Read the model definition and answer for the solid it produces. Units are mm, in the model's axes. A direction names the side the tool comes from. Coordinates: 2 decimals unless noted, no trailing zeros. Write each loop counter-clockwise with the first axis right and the second up, starting at its lowest first coordinate (ties: lowest second). Pieces come first, ordered by that corner, then holes. Notation, with made-up numbers: M -32,55.5 L -14,55.5 A20 ccw -14,59.5 Z; hole C 17.5,-31 d9. An arc over 180 degrees is marked long. Use a Markdown table: item, result. Add a question column.
from build123d import *

# Parameters (mm, degrees)
BOSS_EXTRUDE1_DEPTH = 9.525
CUT_EXTRUDE1_DEPTH  = 19.560809014
SKETCH3_R           = 1.905
CUT_EXTRUDE2_DEPTH  = 19.560809014


with BuildPart() as part:
    # Sketch1 → Boss-Extrude1 (new, symmetric)
    with BuildSketch(Plane.XY):
        with BuildLine():
            Line((6, 0), (6, -10.4775))
            Line((6, -10.4775), (-0.35, -10.4775))
            Line((-0.35, -10.4775), (-5.032019678, -3.267839953))
            ThreePointArc((-5.032019678, -3.267839953), (-1.704095351, 5.752917437), (6, 0))
        make_face()
        Polygon((3.4925, -2.016395815), (3.4925, 2.016395815), (0, 4.03279163), (-3.4925, 2.016395815), (-3.4925, -2.016395815), (0, -4.03279163), align=None, mode=Mode.SUBTRACT)
    extrude(amount=BOSS_EXTRUDE1_DEPTH, both=True)

    # Sketch2 → Cut-Extrude1 (cut, through all)
    with BuildSketch(Plane(origin=(6, 0, 0), x_dir=(0, 0, -1), z_dir=(1, 0, 0))):
        Polygon((-3.175, 6), (-9.525, -6.7), (-9.525, 6), align=None)
    extrude(amount=-CUT_EXTRUDE1_DEPTH, mode=Mode.SUBTRACT)

    # Sketch3 → Cut-Extrude2 (cut, through all)
    with BuildSketch(Plane(origin=(6, 0, 0), x_dir=(0, 0, -1), z_dir=(1, 0, 0))):
        with Locations((-6.35, -7.3025)):
            Circle(SKETCH3_R)
        with Locations((6.35, -7.3025)):
            Circle(SKETCH3_R)
    extrude(amount=-CUT_EXTRUDE2_DEPTH, mode=Mode.SUBTRACT)


solid = part.part
Item 1: For faces 5 (the flat face through (-1.72, 3.04, -2.08)), 6 (the flat face through (2.751, -3.083, 7.717)), determine the directions among +Z, -Z, +X, -X, +Y, -Y from which every point of the face is accessible in a straight line to the end or side of a thin tool.
Item 2: Determine the mould class of faces 1 (the flat face through (-1.77, -3.01, -0.54)), 2 (the flat face through (-3.492, 0, -1)), 3 (the flat face through (3, -10.478, 0)), 4 (the flat face through (-2.66, -6.92, 0.13)) for opening direction X: pulls with the +X half, pulls with the -X half, needs draft (parallel to the pull), parting line crosses it, or undercut.
Item 3: Find section D-D on y = 3.75. Give the vertices of the cut face in (x, z) (3 decimals).
Item 4: Find section B-B on z = -6.35. Give the vertices of the cut face in (x, y).
Item 5: Consider probe 1 along X at (y, z) = (0, 6); probe 2 along Z at (x, y) = (-0.5, -5.75) (3 decimals); probe 3 along Y at (x, z) = (3.25, -6.35). Determine where each line is inside the solid, lowest interval first.
Item 6: Each of these flat-tipped pins is pushed along its axis until it touches: pin 1 (2 mm diameter, centred on x = -4, z = -5.5, fed in from -Y); pin 2 (3 mm diameter, centred on y = 2, z = 2.5, fed in from -X); pin 3 (5 mm diameter, centred on x = 3.5, y = 0.5, fed in from +Z) (3 decimals). Where does it stop, or does it pass through?
Item 7: Find section A-A on x = -0.75. Count the separate pieces of the cut face and the enclosed holes in it, then the cut area to 3 significant figures.
Item 8: Find section C-C on z = 0.5. Give the vertices of the cut face in (x, y), then the cut area to 3 significant figures.
Geometry says:
| question | item | result |
|---|---|---|
| 1 | face 5 | +Z, -Z |
| 1 | face 6 | +Z, +X, -X, +Y |
| 2 | face 1 | undercut |
| 2 | face 2 | undercut |
| 2 | face 3 | needs draft |
| 2 | face 4 | pulls with the -X half |
| 3 | outline | M -4.684,-9.525 L -0.49,-9.525 L -0.49,4.3 L -4.684,4.3 Z; M 0.49,-9.525 L 4.684,-9.525 L 4.684,4.3 L 0.49,4.3 Z |
| 4 | outline | M -5.03,-3.27 L -3.65,-5.4 L 6,-5.4 L 6,0 A6 ccw long Z; M -1.17,-9.21 L -0.35,-10.48 L 6,-10.48 L 6,-9.21 Z; hole M -3.49,-2.02 L 0,-4.03 L 3.49,-2.02 L 3.49,2.02 L 0,4.03 L -3.49,2.02 Z |
| 5 | probe 1 | x = -6 to -3.49, 3.49 to 6 |
| 5 | probe 2 | z = -9.525 to -7.454, -5.246 to 5.246, 7.454 to 9.05 |
| 5 | probe 3 | y = -10.48 to -9.21, -5.4 to -2.16, 2.16 to 5.04 |
| 6 | pin 1 | stops at y = -6.08 |
| 6 | pin 2 | stops at x = -5.98 |
| 6 | pin 3 | stops at z = 7.175 |
| 7 | separate pieces | 2 |
| 7 | enclosed holes | 2 |
| 7 | area | 125 mm2 |
| 8 | outline | M -5.03,-3.27 L -0.35,-10.48 L 6,-10.48 L 6,0 A6 ccw long Z; hole M -3.49,-2.02 L 0,-4.03 L 3.49,-2.02 L 3.49,2.02 L 0,4.03 L -3.49,2.02 Z |
| 8 | area | 115 mm2 |
